Model file for the job. Use its own axes, mm. A direction names the side the tool comes from. Give positions to 0.01 mm unless a question says otherwise; leave off trailing zeros. Order: outer loops, then holes, each group sorted by start corner. A loop starts at its lowest first (then second) coordinate and runs counter-clockwise, first axis right, second up. Notation, with made-up numbers: (37, 18.25) - (81, 18.25) arc R30 ccw to (81, 54.25) - close; hole circle Ø5 at (28, 80.25). An arc over 180 degrees is marked (long way). Return JSON: item names as keys, results as strings. Group by question number.
from build123d import *
from OCP.BRepFilletAPI import BRepFilletAPI_MakeChamfer

# Parameters (mm, degrees)
BOSS_EXTRUDE1_DEPTH = 16
CHAMFER1_SIZE       = 15
CHAMFER1_SIZE2      = 2
SKETCH2_R           = 3
CUT_EXTRUDE1_DEPTH  = 15
CHAMFER2_SIZE       = 2
THREAD1_PITCH       = 1.5
SKETCH5_R           = 7
BOSS_EXTRUDE2_DEPTH = 16
BOSS_EXTRUDE3_START = 10
SKETCH10_W          = 14
SKETCH10_H          = 16
SKETCH10_R          = 3
BOSS_EXTRUDE3_DEPTH = 10
BOSS_EXTRUDE4_START = 10
SKETCH11_R          = 3
BOSS_EXTRUDE4_DEPTH = 10
SKETCH12_R          = 16
CUT_EXTRUDE2_DEPTH  = 7
SKETCH13_R          = 16
BOSS_EXTRUDE5_DEPTH = 9
BOSS_EXTRUDE6_START = -9
BOSS_EXTRUDE6_DEPTH = 9
SKETCH15_R          = 2
CUT_EXTRUDE3_DEPTH  = 20
FILLET1_R           = 5
FILLET2_R           = 5
CUT_EXTRUDE4_START  = -0.5
CUT_EXTRUDE4_DEPTH  = 0.5
SKETCH17_R          = 4
CUT_EXTRUDE5_DEPTH  = 15


with BuildPart() as part:
    # Sketch1 → Boss-Extrude1 (new body)
    with BuildSketch(Plane(origin=(0, 0, 0), x_dir=(0, -1, 0), z_dir=(1, 0, 0))):
        with BuildLine():
            ThreePointArc((-10, 0), (0, 10), (10, 0))
            Line((10, 0), (10, 25))
            Line((10, 25), (-10, 25))
            Line((-10, 25), (-10, 0))
        make_face()
        with BuildLine():
            ThreePointArc((-4.5, 0), (0, 4.5), (4.5, 0))
            Line((4.5, 0), (10, 0))
            ThreePointArc((10, 0), (0, 10), (-10, 0))
            Line((-10, 0), (-4.5, 0))
        make_face()
        with BuildLine():
            Line((10, 0), (4.5, 0))
            ThreePointArc((4.5, 0), (0, -4.5), (-4.5, 0))
            Line((-4.5, 0), (-10, 0))
            ThreePointArc((-10, 0), (0, -10), (10, 0))
        make_face()
    extrude(amount=BOSS_EXTRUDE1_DEPTH)

    # Chamfer1: one chamfer whose edges measure the first distance from different faces: ONE call of the kernel's chamfer builder (chamfer() names one face for all edges)
    chamfer1_edges_1 = [part.edges().sort_by_distance(p)[0] for p in [
        (8, 10, -25),
    ]]
    chamfer1_side_1 = [part.faces().sort_by_distance(p)[0] for p in [
        (8, 10, -12.5),
    ]]
    chamfer1_edges_2 = [part.edges().sort_by_distance(p)[0] for p in [
        (8, -10, -25),
    ]]
    chamfer1_side_2 = [part.faces().sort_by_distance(p)[0] for p in [
        (8, -10, -12.5),
    ]]
    chamfer1_edges_3 = [part.edges().sort_by_distance(p)[0] for p in [
        (16, 0, -25),
    ]]
    chamfer1_side_3 = [part.faces().sort_by_distance(p)[0] for p in [
        (16, 0, -9.408066135),
    ]]
    chamfer1 = BRepFilletAPI_MakeChamfer(part.part.solid().wrapped)
    for e in chamfer1_edges_1:
        chamfer1.Add(CHAMFER1_SIZE, CHAMFER1_SIZE2, e.wrapped, chamfer1_side_1[0].wrapped)  # the first distance lies on this face
    for e in chamfer1_edges_2:
        chamfer1.Add(CHAMFER1_SIZE, CHAMFER1_SIZE2, e.wrapped, chamfer1_side_2[0].wrapped)  # the first distance lies on this face
    for e in chamfer1_edges_3:
        chamfer1.Add(CHAMFER1_SIZE, CHAMFER1_SIZE2, e.wrapped, chamfer1_side_3[0].wrapped)  # the first distance lies on this face
    add(Compound.cast(chamfer1.Shape()), mode=Mode.REPLACE)

    # Sketch2 → Cut-Extrude1 (cut)
    with BuildSketch(Plane(origin=(0, 0, -25), x_dir=(-1, 0, 0), z_dir=(0, 0, -1))):
        with Locations((-8, 0)):
            Circle(SKETCH2_R)
    extrude(amount=-CUT_EXTRUDE1_DEPTH, mode=Mode.SUBTRACT)

    # Chamfer2
    chamfer2_edges = [part.edges().sort_by_distance(p)[0] for p in [
        (0, 0, 10),
        (16, 0, 10),
        (16, 10, -5),
        (0, 10, -5),
        (0, -10, -5),
        (16, -10, -5),
    ]]
    chamfer(chamfer2_edges, length=CHAMFER2_SIZE)

    # Thread1: the profile of Thread Profile1 profile screwed along a right-hand helix of 11.333333 turns, 8 arcs to a turn; built about Z, then put on its axis
    thread1_z = Axis((0, 0, 0), (0, 0, 1))
    thread1_corners = [(4.4997, 0, -0.000173205), (5.311898812, 0, 0.468749998), (5.311898812, 0, 0.656249998), (4.4997, 0, 1.125173201)]
    with BuildLine(mode=Mode.PRIVATE) as thread1_profile:
        Line(thread1_corners[0], thread1_corners[1])
        Line(thread1_corners[1], thread1_corners[2])
        Line(thread1_corners[2], thread1_corners[3])
        Line(thread1_corners[3], thread1_corners[0])
    thread1_cap = Face(thread1_profile.wire())
    thread1_turn_angles = [0, 22.5, 45, 67.5, 90, 112.5, 135, 157.5, 180, 202.5, 225, 247.5, 270, 292.5, 315, 337.5, 360]
    thread1_turn_weights = [1, 0.9238795325112867, 1, 0.9238795325112867, 1, 0.9238795325112867, 1, 0.9238795325112867, 1, 0.9238795325112867, 1, 0.9238795325112867, 1, 0.9238795325112867, 1, 0.9238795325112867, 1]
    thread1_turn_rails = [Edge.make_bspline([Vector(p[0], p[1], 0).rotate(thread1_z, thread1_turn_angles[k]) / thread1_turn_weights[k] + Vector(0, 0, p[2] + THREAD1_PITCH * thread1_turn_angles[k] / 360) for k in range(17)], [0, 0, 0, 1, 1, 2, 2, 3, 3, 4, 4, 5, 5, 6, 6, 7, 7, 8, 8, 8], 2, thread1_turn_weights) for p in thread1_corners]
    thread1_turn_sides = [Face.make_surface_from_curves(thread1_turn_rails[p[0]], thread1_turn_rails[p[1]]) for p in [(0, 1), (1, 2), (2, 3), (3, 0)]]
    thread1_last_angles = [3960, 3982.5, 4005, 4027.5, 4050, 4065, 4080]
    thread1_last_weights = [1, 0.9238795325112867, 1, 0.9238795325112867, 1, 0.9659258262890693, 1]
    thread1_last_rails = [Edge.make_bspline([Vector(p[0], p[1], 0).rotate(thread1_z, thread1_last_angles[k]) / thread1_last_weights[k] + Vector(0, 0, p[2] + THREAD1_PITCH * thread1_last_angles[k] / 360) for k in range(7)], [0, 0, 0, 1, 1, 2, 2, 3, 3, 3], 2, thread1_last_weights) for p in thread1_corners]
    thread1_last_sides = [Face.make_surface_from_curves(thread1_last_rails[p[0]], thread1_last_rails[p[1]]) for p in [(0, 1), (1, 2), (2, 3), (3, 0)]]
    thread1 = Plane(origin=(-1, 0, 0), x_dir=(0, 0, -1), z_dir=(1, 0, 0)) * Solid(Shell([*[p.moved(Location((0, 0, THREAD1_PITCH * i))) for i in range(11) for p in thread1_turn_sides], *thread1_last_sides, thread1_cap, thread1_cap.rotate(thread1_z, 4080).moved(Location((0, 0, THREAD1_PITCH * 4080 / 360)))]))
    add(thread1, mode=Mode.SUBTRACT)

    # Sketch5 → Boss-Extrude2 (add)
    with BuildSketch(Plane.ZY):
        Circle(SKETCH5_R)
    extrude(amount=-BOSS_EXTRUDE2_DEPTH)

    # Sketch10 → Boss-Extrude3 (add)
    with BuildSketch(Plane(origin=(0, 0, -25), x_dir=(-1, 0, 0), z_dir=(0, 0, -1)).offset(BOSS_EXTRUDE3_START)):
        with Locations((-7, 0)):
            Rectangle(SKETCH10_W, SKETCH10_H)
        with Locations((-8, 0)):
            Circle(SKETCH10_R, mode=Mode.SUBTRACT)
    extrude(amount=-BOSS_EXTRUDE3_DEPTH)

    # Sketch11 → Boss-Extrude4 (add)
    with BuildSketch(Plane(origin=(0, 0, -10), x_dir=(-1, 0, 0), z_dir=(0, 0, -1)).offset(BOSS_EXTRUDE4_START)):
        with Locations((-8, 0)):
            Circle(SKETCH11_R)
    extrude(amount=-BOSS_EXTRUDE4_DEPTH)

    # Sketch12 → Cut-Extrude2 (cut)
    with BuildSketch(Plane(origin=(16, 0, 0), x_dir=(0, 0, -1), z_dir=(1, 0, 0))):
        Circle(SKETCH12_R)
    extrude(amount=-CUT_EXTRUDE2_DEPTH, mode=Mode.SUBTRACT)

    # Sketch13 → Boss-Extrude5 (add)
    with BuildSketch(Plane(origin=(9, 0, 0), x_dir=(0, 0, -1), z_dir=(1, 0, 0))):
        Circle(SKETCH13_R)
    extrude(amount=-BOSS_EXTRUDE5_DEPTH)

    # Sketch14 → Boss-Extrude6 (add)
    with BuildSketch(Plane.ZY.offset(BOSS_EXTRUDE6_START)):
        with BuildLine():
            Line((-25, -8), (-13.856406461, -8))
            ThreePointArc((-13.856406461, -8), (-13.341966778, -8.831303556), (-12.777718105, -9.629637586))
            Line((-12.777718105, -9.629637586), (-25, -8))
        make_face()
        with BuildLine():
            Line((-13.856406461, 8), (-25, 8))
            Line((-25, 8), (-12.777718105, 9.629637586))
            ThreePointArc((-12.777718105, 9.629637586), (-13.341966778, 8.831303556), (-13.856406461, 8))
        make_face()
    extrude(amount=BOSS_EXTRUDE6_DEPTH)

    # Sketch15 → Cut-Extrude3 (cut)
    with BuildSketch(Plane(origin=(9, 0, 0), x_dir=(0, 0, -1), z_dir=(1, 0, 0))):
        with Locations((12, 0)):
            Circle(SKETCH15_R)
        with Locations((0, 12)):
            Circle(SKETCH15_R)
        with Locations((-12, 0)):
            Circle(SKETCH15_R)
        with Locations((0, -12)):
            Circle(SKETCH15_R)
    extrude(amount=-CUT_EXTRUDE3_DEPTH, mode=Mode.SUBTRACT)

    # Fillet1
    fillet1_edges = [part.edges().sort_by_distance(p)[0] for p in [
        (4.5, -9.629637586, -12.777718105),
    ]]
    fillet(fillet1_edges, radius=FILLET1_R)

    # Fillet2
    fillet2_edges = [part.edges().sort_by_distance(p)[0] for p in [
        (4.5, 9.629637586, -12.777718105),
    ]]
    fillet(fillet2_edges, radius=FILLET2_R)

    # Sketch16 → Cut-Extrude4 (cut)
    with BuildSketch(Plane.ZY.offset(CUT_EXTRUDE4_START)):
        with BuildLine():
            Line((-14.689269432, 9.374764076), (-25, 8))
            Line((-25, 8), (-35, 8))
            Line((-35, 8), (-35, -8))
            Line((-35, -8), (-25, -8))
            Line((-25, -8), (-14.689269432, -9.374764076))
            ThreePointArc((-14.689269432, -9.374764076), (-13.058341289, -9.887042998), (-11.695305168, -10.918783679))
            ThreePointArc((-11.695305168, -10.918783679), (16, 0), (-11.695305168, 10.918783679))
            ThreePointArc((-11.695305168, 10.918783679), (-13.058341289, 9.887042998), (-14.689269432, 9.374764076))
        make_face()
    extrude(amount=CUT_EXTRUDE4_DEPTH, mode=Mode.SUBTRACT)

    # Sketch17 → Cut-Extrude5 (cut)
    with BuildSketch(Plane(origin=(0, 0, -35), x_dir=(-1, 0, 0), z_dir=(0, 0, -1))):
        with Locations((-8, 0)):
            Circle(SKETCH17_R)
    extrude(amount=-CUT_EXTRUDE5_DEPTH, mode=Mode.SUBTRACT)


solid = part.part
(1) Drop flat-ended pins along their axis: pin 1 Ø10 at (y, z) = (12.5, 6.5) entering from +X; pin 2 Ø6.5 at (x, y) = (8.5, 0) entering from -Z; pin 3 Ø5 at (x, z) = (5, -32.5) entering from +Y; pin 4 Ø3.5 at (y, z) = (-12, 0) entering from +X. Give the stop position or say it passes through.
(2) Slice it at C-C (x = 8). Give the cut face in (y, z), and give its area (3 significant figures).
(3) Slice it at D-D (y = 13). Give the cut face in (x, z), and give its area (3 significant figures).
(4) Drill centre lines: L1, parallel to Y at x = 8, z = -27.25; L2, parallel to X at y = -3, z = -15; L3, parallel to Y at x = 6.5, z = 12. Where is each one in solid material? Low to high.
(5) Slice it at A-A (y = 0). Give the cut face in (x, z).
(6) Pull direction Y, two halves, no side cores. Call faces 1 (the face through (8, 0, -20)), 2 (the face through (7.6, -8.8, -19)), 3 (the face through (5, -10, 0)), 4 (the face through (4.81, 9.876, -13.08)): released by +Y, released by -Y, zero draft, split by the parting line, or undercut.
(7) Slice it at B-B (z = 0). Give the cut face in (x, y).
(8) 3-axis set-ups, long thin cutter, end or side, ignore diameter. For faces 5 (the face through (11.2, -2.4, -27.6)), 6 (the face through (7, -8, -30)), 7 (the face through (7, 8, -30)): which of +Z, -Z, +X, -X, +Y, -Y reach the whole face in a straight line?
Result set:
{
 "1": {"pin 1": "stops at x = 9", "pin 2": "stops at z = -20", "pin 3": "stops at y = 8", "pin 4": "passes through"},
 "2": {"outline": "(-10.92, -11.7) arc R5 cw to (-9.37, -14.69) - (-8, -25) - (-8, -35) - (-4, -35) - (-4, -20) - (4, -20) - (4, -35) - (8, -35) - (8, -25) - (9.37, -14.69) arc R5 cw to (10.92, -11.7) arc R16 ccw (long way) to start; hole circle Ø4 at (-12, 0); hole circle Ø4 at (0, -12); hole circle Ø4 at (0, 12); hole circle Ø4 at (12, 0)", "area": "968 mm²"},
 "3": {"outline": "(0.5, -9.33) - (9, -9.33) - (9, -1.73) - (0.5, -1.73) - close; (0.5, 1.73) - (9, 1.73) - (9, 9.33) - (0.5, 9.33) - close", "area": "129 mm²"},
 "4": {"L1": "y = -8 to -4, 4 to 8", "L2": "x = 0.5 to 9", "L3": "y = -10.58 to -2, 2 to 10.58"},
 "5": {"outline": "(0.5, -35) - (4, -35) - (4, -20) - (12, -20) - (12, -35) - (14, -35) - (14, -25) - (15.2, -16) - (9, -16) - (9, -14) - (0.5, -14) - close; (0.5, -10) - (9, -10) - (9, 10) - (0.5, 10) - close; (0.5, 14) - (9, 14) - (9, 16) - (0.5, 16) - close"},
 "6": {"face 1": "undercut", "face 2": "released by -Y", "face 3": "undercut", "face 4": "released by +Y"},
 "7": {"outline": "(0.5, -16) - (9, -16) - (9, -14) - (0.5, -14) - close; (0.5, -10) - (9, -10) - (9, 10) - (0.5, 10) - close; (0.5, 14) - (9, 14) - (9, 16) - (0.5, 16) - close"},
 "8": {"face 5": "-Z", "face 6": "-Z, +X, -X, -Y", "face 7": "-Z, +X, -X, +Y"}
}
